```python
from build123d import *

# Parameters (mm, degrees)
SKETCH_1_R          = 32.5
EXTRUDE_1_DEPTH     = 27
SKETCH_2_R          = 20
CUT_EXTRUDE_1_DEPTH = 10
CUT_EXTRUDE_2_DEPTH = 6


with BuildPart() as part:
    # 草图1 → 凸台-拉伸1 (new body)
    with BuildSketch(Plane.XY):
        Circle(SKETCH_1_R)
    extrude(amount=EXTRUDE_1_DEPTH)

    # 草图2 → 切除-拉伸1 (cut)
    with BuildSketch(Plane(origin=(0, 0, 0), x_dir=(-1, 0, 0), z_dir=(0, 0, -1))):
        Circle(SKETCH_2_R)
    extrude(amount=-CUT_EXTRUDE_1_DEPTH, mode=Mode.SUBTRACT)

    # 草图3 → 切除-拉伸2 (cut)
    with BuildSketch(Plane(origin=(0, 0, 10), x_dir=(-1, 0, 0), z_dir=(0, 0, -1))):
        Polygon((6, 3.464101615), (0, 6.92820323), (-6, 3.464101615), (-6, -3.464101615), (0, -6.92820323), (6, -3.464101615), align=None)
    extrude(amount=-CUT_EXTRUDE_2_DEPTH, mode=Mode.SUBTRACT)


solid = part.part
```
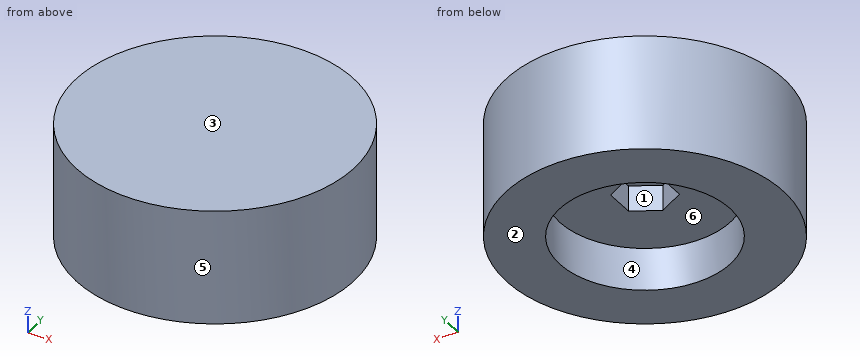
Could you check a few things on this model? Use its own coordinates, in mm. Face numbers are marked on the shaded views. A direction names the side the tool comes from. Round coordinates to 2 decimals unless told otherwise and drop trailing zeros. Write each loop counter-clockwise with the first axis right and the second up, starting at its lowest first coordinate (ties: lowest second). Pieces come first, ordered by that corner, then holes. Notation, with made-up numbers: M -40,-40 L -9,-40 A16 ccw -9,-32 Z; hole C 53,-38 d2. An arc over 180 degrees is marked long. Write each question's results on one line, items separated by ' | '. Start each with the question number.
1. I need wall thicknesses on L1, parallel to Y at x = 0, z = 3; L2, parallel to X at y = 0.5, z = 7.75; L3, parallel to Z at x = -7, y = -1. Which ranges of each line are inside material? Lowest first, please. Write a range as from..to.
2. Imagine slicing it at C-C on x = 5. List the corners of the cut face in (y, z) for me.
3. Imagine slicing it at B-B on y = 0. List the corners of the cut face in (x, z) for me, and give its area (3 significant figures).
4. On a 3-axis mill with a long thin cutter (end or side, diameter ignored), from which of +Z, -Z, +X, -X, +Y, -Y can I reach the whole of each face in a straight line? I mean the marked faces 1 and 2. Say none if no direction works.
5. I'm going to push flat-ended pins straight in: pin 1 Ø4 at (y, z) = (16.5, 19) entering from +X; pin 2 Ø5 at (x, z) = (-1.5, 14) entering from +Y; pin 3 Ø6 at (y, z) = (-14.5, 13) entering from +X. Where does each tip first touch, or does it pass through?
6. Imagine slicing it at A-A on z = 13.5. List the corners of the cut face in (x, y) for me, and give its area (3 significant figures).
7. Thinking about a two-plate mould opening in X: for the marked faces 3, 4, 5 and 6, which applies, +X half, -X half, draft (parallel to the pull), parting line (faces both ways), or undercut?
8. Imagine slicing it at D-D on x = -18. List the corners of the cut face in (y, z) for me.
Result sheet:
1) L1: y = -32.5..-20, 20..32.5 | L2: x = -32.5..-19.99, 19.99..32.5 | L3: z = 10..27
2) outline: M -32.11,0 L -19.36,0 L -19.36,10 L -4.04,10 L -4.04,16 L 4.04,16 L 4.04,10 L 19.36,10 L 19.36,0 L 32.11,0 L 32.11,27 L -32.11,27 Z
3) outline: M -32.5,0 L -20,0 L -20,10 L -6,10 L -6,16 L 6,16 L 6,10 L 20,10 L 20,0 L 32.5,0 L 32.5,27 L -32.5,27 Z | area: 1,280 mm^2
4) face 1: -Z | face 2: -Z, +X, -X, +Y, -Y
5) pin 1: stops at x = 29.09 | pin 2: stops at y = 32.5 | pin 3: stops at x = 30.4
6) outline: C 0,0 d65; hole M -6,-3.46 L 0,-6.93 L 6,-3.46 L 6,3.46 L 0,6.93 L -6,3.46 Z | area: 3,190 mm^2
7) face 3: draft | face 4: undercut | face 5: parting line | face 6: undercut
8) outline: M -27.06,0 L -8.72,0 L -8.72,10 L 8.72,10 L 8.72,0 L 27.06,0 L 27.06,27 L -27.06,27 Z
